Autodesk Inventor part; units mm, degrees
ref_plane "YZ Plane" through (0, 0, 0) normal (1, 0, 0) x (0, 1, 0)
ref_plane "XZ Plane" through (0, 0, 0) normal (0, 1, 0) x (-1, 0, 0)
ref_plane "XY Plane" through (0, 0, 0) normal (0, 0, 1) x (1, 0, 0)
sketch "Эскиз1" plane through (0, 0, 0) normal (1, 0, 0) x (0, 1, 0)
  line L0 (-15.15, 13.4) -> (15.15, 13.4)
  line L1 (15.15, 13.4) -> (15.15, -13.4)
  line L2 (15.15, -13.4) -> (-15.15, -13.4)
  line L3 (-15.15, -13.4) -> (-15.15, 13.4)
  line L4 (-15.15, 13.4) -> (15.15, -13.4) construction
  line L5 (15.15, 13.4) -> (-15.15, -13.4) construction
  point P0 (0, 0)
  dimension "d0" = 30.3
  dimension "d1" = 26.8
extrude "Выдавливание1" add sketch "Эскиз1" along normal blind 8
sketch "Эскиз2" plane through (0, 15.15, 13.4) normal (0, 1, 0) x (1, 0, 0)
  line L0 (4, 2.8) -> (4, 24)
  line L1 (0, 13.4) -> (8, 13.4)
  line L2 (0, 26.8) -> (0, 0)
  line L3 (8, 26.8) -> (8, 0)
  point P0 (0, 13.4)
  point P1 (4, 13.4)
  dimension "d4" = 21.2
hole "Отверстие1" at (4, 15.15, 10.6) at (4, 15.15, -10.6) direction (0, -1, 0) diameter 3.2 end through all
sketch "Эскиз3" plane through (8, 0, 0) normal (1, 0, 0) x (0, 0, -1)
  line L0 (13.4, 15.15) -> (-13.4, 15.15)
  line L1 (-13.4, -15.15) -> (13.4, -15.15)
  line L2 (-13.4, 15.15) -> (13.4, -15.15)
  circle A0 centre (0, 0) radius 5.75
  dimension "d12" = 11.5
extrude "Выдавливание2" cut sketch "Эскиз3" against normal through all
sketch "Эскиз4" plane through (8, 0, 0) normal (1, 0, 0) x (0, 0, -1)
  circle A0 centre (0, 0) radius 5.75
  circle A1 centre (0, 0) radius 7.55
  dimension "d15" = 15.1
extrude "Выдавливание3" cut sketch "Эскиз4" against normal blind 4 contours A0 | A1
properties part number "Differential mount"
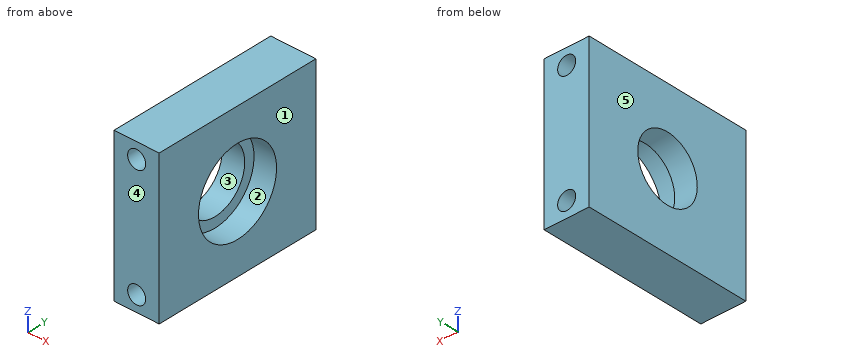
Design review of the part built by this model. Coordinates are the model's own, in mm. Face numbers are marked on the shaded views. A direction names the side the tool comes from. Give positions to 0.01 mm unless a question says otherwise; leave off trailing zeros. Order: outer loops, then holes, each group sorted by start corner. A loop starts at its lowest first (then second) coordinate and runs counter-clockwise, first axis right, second up. Notation, with made-up numbers: (25.25, 87) -> (32.25, 87) arc R34 ccw to (32.25, 121) -> close; hole circle Ø1 at (-29, 48). An arc over 180 degrees is marked (long way). Write item = value, one per line. Start each with the question number.
(1) Mouldability with a two-part tool opening along Y and no side actions: class the marked faces 3, 4 and 5 as +Y half, -Y half, draft (parallel to the pull), parting line (faces both ways), or undercut.
(2) We need section A-A on z = 0. Write out the cut boundary in (x, y), plus the area to 3 significant figures.
(3) For pin 1 (7.5 mm diameter, centred on y = -2.5, z = 2.5, fed in from +X), flat-tipped, find the tip position at first contact; note if it passes through.
(4) To check wall thickness, follow line 1 along Y through (x, z) = (1.6, 0); line 2 along Z through (x, y) = (4.75, -12); line 3 along X through (y, z) = (-3, 10.6). State the ranges of each line that lie inside material, in increasing order.
(5) For the marked faces 1 and 2, list the 3-axis set-ups (+Z, -Z, +X, -X, +Y, -Y) from which the entire face can be reached by the end or side of a thin tool; tool diameter is ignored.
(6) We need section D-D on z = 10.6. Write out the cut boundary in (x, y).
(7) We need section B-B on y = 0. Write out the cut boundary in (x, z).
(8) We need section C-C on x = 7.5. Write out the cut boundary in (y, z), plus the area to 3 significant figures.
Numbers:
q1.face_3 = undercut
q1.face_4 = -Y half
q1.face_5 = draft
q2.outline = (0, -15.15) -> (8, -15.15) -> (8, -7.55) -> (4, -7.55) -> (4, -5.75) -> (0, -5.75) -> close; (0, 5.75) -> (4, 5.75) -> (4, 7.55) -> (8, 7.55) -> (8, 15.15) -> (0, 15.15) -> close
q2.area = 136 mm^2
q3.pin_1 = 4
q4.line_1 = -15.15 to -5.75, 5.75 to 15.15
q4.line_2 = -13.4 to -12.01, -9.19 to 9.19, 12.01 to 13.4
q4.line_3 = 0 to 2.4, 5.6 to 8
q5.face_1 = +Z, -Z, +X, +Y, -Y
q5.face_2 = +X
q6.outline = (0, -15.15) -> (2.4, -15.15) -> (2.4, 15.15) -> (0, 15.15) -> close; (5.6, -15.15) -> (8, -15.15) -> (8, 15.15) -> (5.6, 15.15) -> close
q7.outline = (0, -13.4) -> (8, -13.4) -> (8, -7.55) -> (4, -7.55) -> (4, -5.75) -> (0, -5.75) -> close; (0, 5.75) -> (4, 5.75) -> (4, 7.55) -> (8, 7.55) -> (8, 13.4) -> (0, 13.4) -> close; hole circle Ø3.2 at (4, -10.6); hole circle Ø3.2 at (4, 10.6)
q8.outline = (-15.15, -13.4) -> (15.15, -13.4) -> (15.15, 13.4) -> (-15.15, 13.4) -> close; hole circle Ø15.1 at (0, 0)
q8.area = 633 mm^2
